Geometry: final body of the model. Coordinates: model frame, mm. Coordinates: 2 decimals unless noted, no trailing zeros. Write each loop counter-clockwise with the first axis right and the second up, starting at its lowest first coordinate (ties: lowest second). Pieces come first, ordered by that corner, then holes. Notation, with made-up numbers: M 39,74.25 L 98,74.25 A9 cw 98,80.25 Z; hole C -13.5,50.25 d7. An arc over 180 degrees is marked long. Write item = value, one per line. Start each with the question number.
Item 1: Section B-B on z = 70. Output: boundary loops of the cut face in (x, y), plus the area to 3 significant figures.
Item 2: Ray query, L1, parallel to X at y = 2.45, z = -70; L2, parallel to Z at x = -45, y = 1.4; L3, parallel to Z at x = -44.5, y = 3.25. Return the intervals inside material, ascending. Write a range as [from, to].
Item 3: Section A-A on x = -45. Output: boundary loops of the cut face in (y, z).
Item 4: Pull-direction query (Z, two-part tool) for faces 1 (the flat face through (-1, 0, -1)), 2 (the cylindrical face through (42.56, 2.54, 69.46)), 3 (the cylindrical face through (-0.66, 4.1, -74.14)); classes: +Z half, -Z half, draft (parallel to the pull), parting line (faces both ways), or undercut.
from build123d import *

# Parameters (mm, degrees)
SKETCH1_W           = 100
SKETCH1_H           = 150
BOSS_EXTRUDE1_DEPTH = 5
SKETCH2_R           = 2.5
CUT_EXTRUDE1_DEPTH  = 91.277350426
FILLET1_R           = 3


with BuildPart() as part:
    # Sketch1 → Boss-Extrude1 (new body)
    with BuildSketch(Plane(origin=(0, 0, 0), x_dir=(1, 0, 0), z_dir=(0, 1, 0))):
        Rectangle(SKETCH1_W, SKETCH1_H)
    extrude(amount=BOSS_EXTRUDE1_DEPTH)

    # Sketch2 → Cut-Extrude1 (cut, through all)
    with BuildSketch(Plane(origin=(0, 5, 0), x_dir=(1, 0, 0), z_dir=(0, 1, 0))):
        with Locations(Location((-45, 70, 0), (0, 0, 270))):
            Circle(SKETCH2_R)
        with Locations(Location((45, 70, 0), (0, 0, 90))):
            Circle(SKETCH2_R)
        with Locations(Location((45, -70, 0), (0, 0, 270))):
            Circle(SKETCH2_R)
        with Locations(Location((-45, -70, 0), (0, 0, 90))):
            Circle(SKETCH2_R)
    extrude(amount=-CUT_EXTRUDE1_DEPTH, mode=Mode.SUBTRACT)

    # Fillet1
    # the kernel refuses this fillet: 3 mm, written as the material it takes off along each edge
    with BuildSketch(Plane(origin=(-47, 2, -72), x_dir=(-1, 0, 0), z_dir=(0, 0, -1))) as fillet1_piece_1_section:
        Polygon((0, 0), (FILLET1_R, 0), (FILLET1_R, FILLET1_R), (0, FILLET1_R), align=None)
    fillet1_piece_1 = extrude(amount=FILLET1_R, mode=Mode.PRIVATE)
    fillet1_piece_1 = fillet1_piece_1 - Plane(origin=(-47, 2, -72), x_dir=(0.7071067811865475, -0.7071067811865475, 0), z_dir=(0, 0, -1)) * Sphere(FILLET1_R, mode=Mode.PRIVATE)
    add(fillet1_piece_1, mode=Mode.SUBTRACT)
    with BuildSketch(Plane(origin=(47, 2, -72), x_dir=(1, 0, 0), z_dir=(0, 0, -1))) as fillet1_piece_2_section:
        Polygon((0, 0), (FILLET1_R, 0), (FILLET1_R, -FILLET1_R), (0, -FILLET1_R), align=None)
    fillet1_piece_2 = extrude(amount=FILLET1_R, mode=Mode.PRIVATE)
    fillet1_piece_2 = fillet1_piece_2 - Plane(origin=(47, 2, -72), x_dir=(-0.7071067811865475, -0.7071067811865475, 0), z_dir=(0, 0, -1)) * Sphere(FILLET1_R, mode=Mode.PRIVATE)
    add(fillet1_piece_2, mode=Mode.SUBTRACT)
    with BuildSketch(Plane(origin=(-50, 5, 82.5), x_dir=(0, -1, 0), z_dir=(0, 0, -1)), Plane(origin=(50, 5, -72), x_dir=(0, -1, 0), z_dir=(0, 0, 1))) as fillet1_piece_3:
        with BuildLine():
            CenterArc((FILLET1_R, -FILLET1_R), FILLET1_R, 90, 90)
            Line((0, -FILLET1_R), (0, 0))
            Line((0, 0), (FILLET1_R, 0))
        make_face()
    extrude(amount=154.5, mode=Mode.SUBTRACT)
    with BuildSketch(Plane(origin=(-50, -7.5, -75), x_dir=(1, 0, 0), z_dir=(0, 1, 0))) as fillet1_piece_4:
        with BuildLine():
            CenterArc((FILLET1_R, -FILLET1_R), FILLET1_R, 90, 90)
            Line((0, -FILLET1_R), (0, 0))
            Line((0, 0), (FILLET1_R, 0))
        make_face()
    extrude(amount=9.5, mode=Mode.SUBTRACT)
    with BuildSketch(Plane(origin=(50, -7.5, -75), x_dir=(-1, 0, 0), z_dir=(0, 1, 0))) as fillet1_piece_5:
        with BuildLine():
            CenterArc((FILLET1_R, FILLET1_R), FILLET1_R, 180, 90)
            Line((0, FILLET1_R), (0, 0))
            Line((0, 0), (FILLET1_R, 0))
        make_face()
    extrude(amount=9.5, mode=Mode.SUBTRACT)
    with BuildSketch(Plane(origin=(-47, 5, -75), x_dir=(0, -1, 0), z_dir=(1, 0, 0))) as fillet1_piece_6:
        with BuildLine():
            CenterArc((FILLET1_R, -FILLET1_R), FILLET1_R, 90, 90)
            Line((0, -FILLET1_R), (0, 0))
            Line((0, 0), (FILLET1_R, 0))
        make_face()
    extrude(amount=94, mode=Mode.SUBTRACT)


solid = part.part
Responses:
q1.outline = M -50,0 L -47.5,0 L -47.5,4.96 A3 ccw -50,2 Z; M -42.5,0 L 42.5,0 L 42.5,5 L -42.5,5 Z; M 47.5,0 L 50,0 L 50,2 A3 ccw 47.5,4.96 Z
q1.area = 446 mm²
q2.L1 = [-49.97, -47.5], [-42.5, 42.5], [47.5, 49.97]
q2.L2 = [-75, -72.5], [-67.5, 67.5], [72.5, 75]
q2.L3 = [-74.73, -72.45], [-67.55, 67.55], [72.45, 75]
q3.outline = M 0,-75 L 2,-75 A3 ccw 4.96,-72.5 L 0,-72.5 Z; M 0,-67.5 L 5,-67.5 L 5,67.5 L 0,67.5 Z; M 0,72.5 L 5,72.5 L 5,75 L 0,75 Z
q4.face_1 = draft
q4.face_2 = undercut
q4.face_3 = -Z half
